from build123d import *

# Parameters (mm, degrees)
F0_R     = 1
F1_DEPTH = 1.5


with BuildPart() as f1:
    # F0 (on Front) → F1 (new body, symmetric)
    with BuildSketch(Plane.XZ):
        Polygon((-20, 0), (0, 0), (0, 7), (3, 7), (3, 17), (0, 17), (0, 24), (3, 24), (3, 34), (0, 34), (0, 41), (-20, 41), (-20, 38), (-30, 38), (-30, 41), (-50, 41), (-50, 38), (-60, 38), (-60, 41), (-80, 41), (-80, 38), (-84, 38), (-84, 33), (-83, 33), (-83, 31), (-84, 31), (-84, 26), (-86, 26), (-86, 31), (-87, 31), (-87, 33), (-86, 33), (-86, 38), (-90, 38), (-90, 41), (-110, 41), (-110, 34), (-113, 34), (-113, 24), (-110, 24), (-110, 17), (-113, 17), (-113, 7), (-110, 7), (-110, 0), (-90, 0), (-90, 3), (-80, 3), (-80, 0), (-60, 0), (-60, 3), (-50, 3), (-50, 0), (-30, 0), (-30, 3), (-20, 3), align=None)
        with Locations((-70, 1.5)):
            Circle(F0_R, mode=Mode.SUBTRACT)
        with Locations((-40, 1.5)):
            Circle(F0_R, mode=Mode.SUBTRACT)
        with Locations((-70, 39.5)):
            Circle(F0_R, mode=Mode.SUBTRACT)
        with Locations((-40, 39.5)):
            Circle(F0_R, mode=Mode.SUBTRACT)
    extrude(amount=F1_DEPTH, both=True)


solid = f1.part
Here's how the part is built. I have some questions about the finished solid (model axes, mm). A direction names the side the tool comes from. Coordinates: 2 decimals unless noted, no trailing zeros. Write each loop counter-clockwise with the first axis right and the second up, starting at its lowest first coordinate (ties: lowest second). Pieces come first, ordered by that corner, then holes.
1) Which directions (+Z, -Z, +X, -X, +Y, -Y) give clear straight access to the entire face, cutting with the end or side of a thin tool? Please do faces 4 (the face through (-86, 0, 35)), 5 (the face through (-112, 0, 7)), 6 (the face through (0, 0, 3)).
Filled in:
face 4: +Z, +Y, -Y
face 5: -Z, -X, +Y, -Y
face 6: -Z, +X, +Y, -Y
2) If we section it at C-C (y = 0.7): Count the separate pieces of the cut face and the enclosed holes in it, plus the area to 3 significant figures.
Filled in:
separate pieces: 1
enclosed holes: 4
area: 4,410 mm2
3) Thinking about a two-plate mould opening in Z: for faces 1 (the face through (-82, 0, 38)), 2 (the face through (0, 0, 37)), 3 (the face through (-111, 0, 17)), which applies, +Z half, -Z half, draft (parallel to the pull), parting line (faces both ways), or undercut?
Filled in:
face 1: +Z half
face 2: draft
face 3: undercut
4) If we section it at B-B (z = 1.5): List the corners of the cut face in (x, y) for me, plus the area to 3 significant figures.
Filled in:
outline: (-110, -1.5) - (-90, -1.5) - (-90, 1.5) - (-110, 1.5) - close; (-80, -1.5) - (-71, -1.5) - (-71, 1.5) - (-80, 1.5) - close; (-69, -1.5) - (-60, -1.5) - (-60, 1.5) - (-69, 1.5) - close; (-50, -1.5) - (-41, -1.5) - (-41, 1.5) - (-50, 1.5) - close; (-39, -1.5) - (-30, -1.5) - (-30, 1.5) - (-39, 1.5) - close; (-20, -1.5) - (0, -1.5) - (0, 1.5) - (-20, 1.5) - close
area: 228 mm2
5) If we section it at D-D (x = -59): List the corners of the cut face in (y, z) for me.
Filled in:
outline: (-1.5, 3) - (1.5, 3) - (1.5, 38) - (-1.5, 38) - close
6) If we section it at A-A (x = -40): List the corners of the cut face in (y, z) for me, plus the area to 3 significant figures.
Filled in:
outline: (-1.5, 0) - (1.5, 0) - (1.5, 0.5) - (-1.5, 0.5) - close; (-1.5, 2.5) - (1.5, 2.5) - (1.5, 38.5) - (-1.5, 38.5) - close; (-1.5, 40.5) - (1.5, 40.5) - (1.5, 41) - (-1.5, 41) - close
area: 111 mm2
7) I'm going to push flat-ended pins straight in: pin 1 (0.9 mm diameter, centred on x = -112, y = 0.5, fed in from +Z); pin 2 (1.8 mm diameter, centred on x = -40, z = 39.5, fed in from +Y); pin 3 (0.9 mm diameter, centred on x = -111.5, y = 0.5, fed in from -Z); pin 4 (1.5 mm diameter, centred on x = -81, y = 0.5, fed in from -Z). Where does each tip first touch, or does it pass through?
Filled in:
pin 1: stops at z = 34
pin 2: passes through
pin 3: stops at z = 7
pin 4: stops at z = 3
8) If I drill on line 1 (Z direction, x = -40, y = -0.85); line 2 (X direction, y = 1.15, z = 30.5); line 3 (X direction, y = 0.5, z = 20.5), over which ranges is the centre line in solid material (lowest first)?
Filled in:
line 1: z = 0 to 0.5, 2.5 to 38.5, 40.5 to 41
line 2: x = -113 to -86, -84 to 3
line 3: x = -110 to 0
